```python
from build123d import *

# Parameters (mm, degrees)
F3_R     = 4
F4_DEPTH = 128
F5_R     = 8
F6_DEPTH = 20


with BuildPart() as f1:
    # F0 (on Front) → F1 (revolve)
    with BuildSketch(Plane.XZ):
        with BuildLine():
            Line((-30, 0), (0, 0))
            Line((0, 0), (0, 74.4419768453))
            add(Edge.make_bspline(
                [(-30, 0), (-26.0781444115, 13.4116450928), (-18.4118492623, 39.6282222706), (-76.4407572251, 59.6656107835), (-13.1944315406, 79.611542342), (-3.5713194359, 75.8412163409), (0, 74.4419768453)],
                knots=[0, 0, 0, 0, 0.2714940232, 0.5307062604, 0.8258361915, 1, 1, 1, 1], degree=3))
        make_face()
    revolve(axis=Axis((0, 0, 37.2209884226), (0, 0, 1)))

    # F3 (on offset) → F4 (cut)
    with BuildSketch(Plane.XY.offset(82)):
        Circle(F3_R)
    extrude(amount=-F4_DEPTH, mode=Mode.SUBTRACT)

    # F5 (on offset) → F6 (cut)
    with BuildSketch(Plane.XY.offset(82)):
        Circle(F5_R)
    extrude(amount=-F6_DEPTH, mode=Mode.SUBTRACT)


solid = f1.part
```
The model under review builds one solid part; all positions refer to its coordinate system, in mm. A direction names the side the tool comes from. Give positions to 0.01 mm unless a question says otherwise; leave off trailing zeros. Answer in a Markdown table with one row per item.
1) Mouldability with a two-part tool opening along X and no side actions: class faces 3 (the flat face through (0, 6, 0)), 4 (the flat face through (-4, -2, 62)) as +X half, -X half, draft (parallel to the pull), parting line (faces both ways), or undercut.
Worked answers:
| item | result |
|---|---|
| face 3 | draft |
| face 4 | undercut |
2) Clearance check with flat-ended pins moving along their axes: P1, Ø1.5, axis at x = -29, z = 50.5, coming from the -Y side; P2, Ø12, axis at y = 24, z = 31.5, coming from the +X side; P3, Ø3, axis at x = 41, y = 11.5, coming from the -Z side. State where each tip first meets the part, or that it passes through.
Worked answers:
| item | result |
|---|---|
| P1 | y = -39.37 |
| P2 | x = 21.58 |
| P3 | z = 46.05 |
3) For L1, parallel to Y at x = 0, z = 17.5; L2, parallel to Y at x = 0, z = 15; L3, parallel to X at y = 0, z = 67, list the stretches that pass through material, from the lowest coordinate up. Write a range as [from, to].
Worked answers:
| item | result |
|---|---|
| L1 | [-25.81, -4], [4, 25.81] |
| L2 | [-26.19, -4], [4, 26.19] |
| L3 | [-46.44, -8], [8, 46.44] |
4) Tool access review of faces 1 (the cylindrical face through (-1.73, -7.81, 69.37)), 2 (the cylindrical face through (-0.867, -3.905, 31.434)): name each direction out of +Z, -Z, +X, -X, +Y, -Y from which nothing blocks a thin tool from reaching the whole face with its end or side.
Worked answers:
| item | result |
|---|---|
| face 1 | +Z |
| face 2 | +Z, -Z |
